Can you work these out from the model? Positions are in its coordinate system, mm. Face numbers are marked on the shaded views. A direction names the side the tool comes from. Round coordinates to 2 decimals unless told otherwise and drop trailing zeros. Loops run counter-clockwise (first coordinate to the right, second up) from the corner with the lowest first, then second, coordinate; pieces in that order, holes last. Notation, with made-up numbers: (-18, 88.5) -> (33, 88.5) arc R12 ccw to (33, 102.5) -> close; hole circle Ø3 at (-25.5, 4). An arc over 180 degrees is marked (long way). Use a Markdown table: item, result.
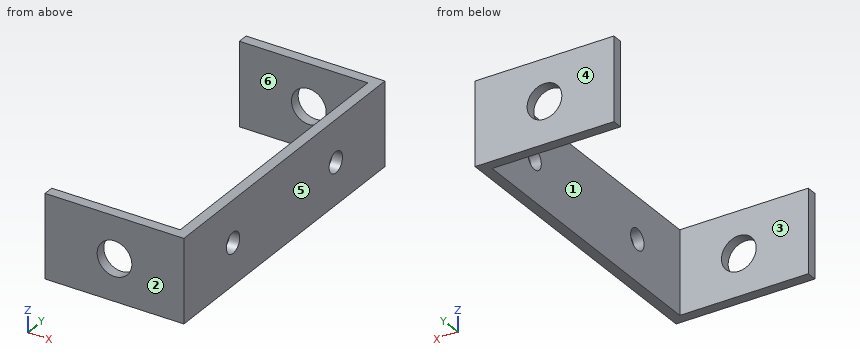
from build123d import *

# Parameters (mm, degrees)
SKETCH1_W           = 18.5
SKETCH1_H           = 12
BOSS_EXTRUDE1_DEPTH = 1.5
SKETCH1_3_W         = 1.5
SKETCH1_3_H         = 12
BOSS_EXTRUDE2_DEPTH = 45
SKETCH2_R           = 1.5
CUT_EXTRUDE1_DEPTH  = 50.608467019
BOSS_EXTRUDE3_START = -45
SKETCH1_4_W         = 18.5
SKETCH1_4_H         = 12
BOSS_EXTRUDE3_DEPTH = 1.5
SKETCH3_R           = 2.5
CUT_EXTRUDE2_DEPTH  = 47.486557197


with BuildPart() as part:
    # Sketch1 → Boss-Extrude1 (new body)
    with BuildSketch(Plane(origin=(0, 0, 0), x_dir=(1, 0, 0), z_dir=(0, 1, 0))):
        with Locations((-0.75, 0)):
            Rectangle(SKETCH1_W, SKETCH1_H)
    extrude(amount=-BOSS_EXTRUDE1_DEPTH)

    # Sketch1<3> → Boss-Extrude2 (add)
    with BuildSketch(Plane(origin=(0, 0, 0), x_dir=(1, 0, 0), z_dir=(0, 1, 0))):
        with Locations((9.25, 0)):
            Rectangle(SKETCH1_3_W, SKETCH1_3_H)
    extrude(amount=-BOSS_EXTRUDE2_DEPTH)

    # Sketch2 → Cut-Extrude1 (cut, through all)
    with BuildSketch(Plane(origin=(10, 0, 0), x_dir=(0, 0, -1), z_dir=(1, 0, 0))):
        with Locations((0, -34)):
            Circle(SKETCH2_R)
        with Locations((0, -11)):
            Circle(SKETCH2_R)
    extrude(amount=-CUT_EXTRUDE1_DEPTH, mode=Mode.SUBTRACT)

    # Sketch1<4> → Boss-Extrude3 (add)
    with BuildSketch(Plane(origin=(0, 0, 0), x_dir=(1, 0, 0), z_dir=(0, 1, 0)).offset(BOSS_EXTRUDE3_START)):
        with Locations((-0.75, 0)):
            Rectangle(SKETCH1_4_W, SKETCH1_4_H)
    extrude(amount=BOSS_EXTRUDE3_DEPTH)

    # Sketch3 → Cut-Extrude2 (cut, through all)
    with BuildSketch(Plane(origin=(0, 0, 0), x_dir=(1, 0, 0), z_dir=(0, 1, 0))):
        with Locations(Location((0, 0, 0), (0, 0, 270))):
            Circle(SKETCH3_R)
    extrude(amount=-CUT_EXTRUDE2_DEPTH, mode=Mode.SUBTRACT)


solid = part.part
1. I want a section at C-C (y = -11). Please give me the cut outline in (x, z).
Answer sheet:
| item | result |
|---|---|
| outline | (8.5, -6) -> (10, -6) -> (10, -1.5) -> (8.5, -1.5) -> close; (8.5, 1.5) -> (10, 1.5) -> (10, 6) -> (8.5, 6) -> close |
2. I want a section at B-B (z = 2). Please give me the cut outline in (x, y).
Answer sheet:
| item | result |
|---|---|
| outline | (-10, -45) -> (-1.5, -45) -> (-1.5, -43.5) -> (-10, -43.5) -> close; (-10, -1.5) -> (-1.5, -1.5) -> (-1.5, 0) -> (-10, 0) -> close; (1.5, -45) -> (10, -45) -> (10, 0) -> (1.5, 0) -> (1.5, -1.5) -> (8.5, -1.5) -> (8.5, -43.5) -> (1.5, -43.5) -> close |
3. I want a section at D-D (z = 0). Please give me the cut outline in (x, y).
Answer sheet:
| item | result |
|---|---|
| outline | (-10, -45) -> (-2.5, -45) -> (-2.5, -43.5) -> (-10, -43.5) -> close; (-10, -1.5) -> (-2.5, -1.5) -> (-2.5, 0) -> (-10, 0) -> close; (2.5, -45) -> (10, -45) -> (10, -35.5) -> (8.5, -35.5) -> (8.5, -43.5) -> (2.5, -43.5) -> close; (2.5, -1.5) -> (8.5, -1.5) -> (8.5, -9.5) -> (10, -9.5) -> (10, 0) -> (2.5, 0) -> close; (8.5, -32.5) -> (10, -32.5) -> (10, -12.5) -> (8.5, -12.5) -> close |
4. Will these pins go through, and if not, where does the flat tip stop? pin 1 Ø3 at (x, z) = (0, 0) entering from -Y; pin 2 Ø3.5 at (y, z) = (-11, 0) entering from -X; pin 3 Ø6 at (x, z) = (3, 2.5) entering from +Y.
Answer sheet:
| item | result |
|---|---|
| pin 1 | passes through |
| pin 2 | stops at x = 8.5 |
| pin 3 | stops at y = 0 |
5. If we mould it in two halves opening along Y, with no side actions, what happens to the marked faces 3, 4, 5 and 6? For each: +Y half, -Y half, draft (parallel to the pull), parting line (faces both ways), or undercut.
Answer sheet:
| item | result |
|---|---|
| face 3 | undercut |
| face 4 | +Y half |
| face 5 | draft |
| face 6 | undercut |
6. Which directions (+Z, -Z, +X, -X, +Y, -Y) give clear straight access to the entire face, cutting with the end or side of a thin tool? Please do the marked faces 1 and 2.
Answer sheet:
| item | result |
|---|---|
| face 1 | +Z, -Z, -X |
| face 2 | +Z, -Z, +X, -X, -Y |
7. I need wall thicknesses on line 1 (Y direction, x = -4.75, z = -4.5); line 2 (X direction, y = -44.4, z = 0); line 3 (X direction, y = -24, z = 4.5). Which ranges of each line are inside material? Lowest first, please.
Answer sheet:
| item | result |
|---|---|
| line 1 | y = -45 to -43.5, -1.5 to 0 |
| line 2 | x = -10 to -2.5, 2.5 to 10 |
| line 3 | x = 8.5 to 10 |
8. I want a section at A-A (x = 0). Please give me the cut outline in (y, z).
Answer sheet:
| item | result |
|---|---|
| outline | (-45, -6) -> (-43.5, -6) -> (-43.5, -2.5) -> (-45, -2.5) -> close; (-45, 2.5) -> (-43.5, 2.5) -> (-43.5, 6) -> (-45, 6) -> close; (-1.5, -6) -> (0, -6) -> (0, -2.5) -> (-1.5, -2.5) -> close; (-1.5, 2.5) -> (0, 2.5) -> (0, 6) -> (-1.5, 6) -> close |
